Source: CAD feature listing. Evaluate the final solid. Frame: model axes, mm. A direction names the side the tool comes from. Coordinates: 2 decimals unless noted, no trailing zeros. Order: outer loops, then holes, each group sorted by start corner. A loop starts at its lowest first (then second) coordinate and runs counter-clockwise, first axis right, second up. Notation, with made-up numbers: (17.5, 27.5) - (58.5, 27.5) arc R31 cw to (58.5, 60.5) - close; hole circle Ø3 at (84.25, 88.5). An arc over 180 degrees is marked (long way). One line per question, with ' | ' between items. Start each with the question number.
(1) Draft query along X for faces 1 (the flat face through (25, -28, 2)), 2 (the flat face through (0, -14, 4)), 3 (the cylindrical face through (46.364, -15.187, 3.944)), 4 (the cylindrical face through (25, -14, -12)). Return one class per face: +X half, -X half, draft (parallel to the pull), parting line (faces both ways), or undercut.
(2) Line query: line 1 along Y through (x, z) = (6.5, 6.25); line 2 along X through (y, z) = (-7.75, -0.5); line 3 along Z through (x, y) = (43, -18.5). Output: solid intervals per line, ascending.
(3) Section C-C (z = -9.5). Return the cut outline in (x, y).
(4) Section B-B (x = 43.5). Return the cut outline in (y, z).
(5) Access query for faces 5 (the flat face through (6.4, -10.7, 0)), 6 (the flat face through (25, 0, 2)), 7 (the flat face through (43.4, -10.7, 0)). Directions: +Z, -Z, +X, -X, +Y, -Y. A direction counts if a zero-diameter tool reaches every point of the face in a straight line with its end or side. Return the directions, or none.
(6) Section A-A (y = -14). Return the cut outline in (x, z).
(7) Contact query for flat-ended pins moving along their axis: P1, Ø3, axis at y = -18.5, z = -4.5, coming from the +X side; P2, Ø6.5, axis at x = 40.5, y = -18.5, coming from the -Z side; P3, Ø1, axis at x = 13.5, y = -6, coming from the -Z side; P4, Ø4, axis at y = -18, z = 2, coming from the -X side. Output: stop coordinate, or through.
(8) Section D-D (y = -8.25). Return the cut outline in (x, z), then the cut area to 3 significant figures.
from build123d import *

# Parameters (mm, degrees)
SKETCH_1_W          = 50
SKETCH_1_H          = 28
EXTRUDE_1_DEPTH     = 8
EXTRUDE_2_DEPTH     = 28
CUT_EXTRUDE_1_DEPTH = 28
SKETCH_1_4_R        = 3.1
CUT_EXTRUDE_2_DEPTH = 8


with BuildPart() as part:
    # 草图1 → 凸台-拉伸1 (new body)
    with BuildSketch(Plane.XY):
        with Locations((25, -14)):
            Rectangle(SKETCH_1_W, SKETCH_1_H)
    extrude(amount=EXTRUDE_1_DEPTH)

    # 草图2 → 凸台-拉伸2 (add)
    with BuildSketch(Plane.XZ.offset(28)):
        with BuildLine():
            Line((37, 0), (25, 0))
            Line((25, 0), (13, 0))
            ThreePointArc((13, 0), (25, -12), (37, 0))
        make_face()
    extrude(amount=-EXTRUDE_2_DEPTH)

    # 草图3 → 切除-拉伸1 (cut)
    with BuildSketch(Plane.XZ.offset(28)):
        with BuildLine():
            ThreePointArc((25, -2), (21, -6), (25, -10))
            Line((25, -10), (25, -2))
        make_face()
        with BuildLine():
            Line((25, -2), (25, -10))
            ThreePointArc((25, -10), (27.828427125, -8.828427125), (29, -6))
            ThreePointArc((29, -6), (27.828427125, -3.171572875), (25, -2))
        make_face()
    extrude(amount=-CUT_EXTRUDE_1_DEPTH, mode=Mode.SUBTRACT)

    # 草图1<4> → 切除-拉伸2 (cut)
    with BuildSketch(Plane.XY):
        with Locations((6.5, -14)):
            Circle(SKETCH_1_4_R)
        with Locations((43.5, -14)):
            Circle(SKETCH_1_4_R)
    extrude(amount=CUT_EXTRUDE_2_DEPTH, mode=Mode.SUBTRACT)


solid = part.part
Response values:
1) face 1: draft | face 2: -X half | face 3: undercut | face 4: parting line
2) line 1: y = -28 to -17.1, -10.9 to 0 | line 2: x = 13.01 to 36.99 | line 3: z = 0 to 8
3) outline: (17.67, -28) - (23.06, -28) - (23.06, 0) - (17.67, 0) - close; (26.94, -28) - (32.33, -28) - (32.33, 0) - (26.94, 0) - close
4) outline: (-28, 0) - (-17.1, 0) - (-17.1, 8) - (-28, 8) - close; (-10.9, 0) - (0, 0) - (0, 8) - (-10.9, 8) - close
5) face 5: -Z, -X, +Y, -Y | face 6: +Z, -Z, +X, -X, +Y | face 7: -Z, +X, +Y, -Y
6) outline: (0, 0) - (3.4, 0) - (3.4, 8) - (0, 8) - close; (9.6, 0) - (13, 0) arc R12 ccw to (37, 0) - (40.4, 0) - (40.4, 8) - (9.6, 8) - close; (46.6, 0) - (50, 0) - (50, 8) - (46.6, 8) - close; hole circle Ø8 at (25, -6)
7) P1: stops at x = 36.62 | P2: stops at z = 0 | P3: stops at z = -4.8 | P4: stops at x = 0
8) outline: (0, 0) - (13, 0) arc R12 ccw to (37, 0) - (50, 0) - (50, 8) - (0, 8) - close; hole circle Ø8 at (25, -6) | area: 576 mm²
